Can you work these out from the model? Positions are in its coordinate system, mm. A direction names the side the tool comes from. Round coordinates to 2 decimals unless told otherwise and drop trailing zeros. Write each loop counter-clockwise with the first axis right and the second up, starting at its lowest first coordinate (ties: lowest second). Pieces come first, ordered by that corner, then holes. Notation, with made-up numbers: (19.5, -38.5) - (44.5, -38.5) arc R23 cw to (44.5, -18.5) - close; hole circle Ø2 at (-10, -29.5). An arc over 180 degrees is marked (long way). One line per item, written item: value. Start each with the question number.
(1) I want a section at A-A on z = 15.5. List the corners of the cut face in (x, y) for me (3 decimals).
(2) I want a section at C-C on x = 0. List the corners of the cut face in (y, z) for me, plus the area to 3 significant figures.
(3) Thinking about a two-plate mould opening in X: for faces 5 (the face through (32.96, 11.524, 18.645)), 6 (the face through (16, 30, 25)), 7 (the face through (26.46, -22.78, 18.64)), which applies, +X half, -X half, draft (parallel to the pull), parting line (faces both ways), or undercut?
(4) If I drill on L1, parallel to X at y = 0, z = 19.25; L2, parallel to X at y = 3.5, z = 6.5, over which ranges is the centre line in solid material (lowest first)? Write a range as from..to.
(5) I'm going to push flat-ended pins straight in: pin 1 Ø1 at (x, z) = (-8, 6.5) entering from -Y; pin 2 Ø8.5 at (x, y) = (-1.5, 34) entering from +Z; pin 3 Ø1.5 at (x, y) = (27.5, 6.5) entering from +Z. Where does each tip first touch, or does it pass through?
(6) On a 3-axis mill with a long thin cutter (end or side, diameter ignored), from which of +Z, -Z, +X, -X, +Y, -Y can I reach the whole of each face in a straight line? I mean faces 1 (the face through (0, 35, 12.109)), 2 (the face through (-26.46, 22.78, 18.64)), 3 (the face through (-33.084, 11.595, 18.645)), 4 (the face through (26.58, 22.85, 18.64)). Say none if no direction works.
(7) I want a section at B-B on y = 0. List the corners of the cut face in (x, z) for me, plus the area to 3 significant figures.
(8) I want a section at D-D on z = -1.5. List the corners of the cut face in (x, y) for me.
from build123d import *

# Parameters (mm, degrees)
F0_R            = 40
F0_R_2          = 30
F1_DEPTH        = 25
F3_DEPTH        = 12.8905829042
F3_COPIES_COUNT = 6
F5_R            = 40
F5_R_2          = 30
F6_DEPTH        = 5.8128256351


# Not quite as in the source:
# - a pattern or mirror of a feature is missing from the dataset's text; its kind, count and spacing are read off the source's solid


with BuildPart() as f1:
    # F0 (on Top) → F1 (new body)
    with BuildSketch(Plane.XY):
        Circle(F0_R)
        Circle(F0_R_2, mode=Mode.SUBTRACT)
    extrude(amount=F1_DEPTH)

    # F2 (on face) → F3 (cut)
    with BuildSketch(Plane.XY.offset(25)):
        with BuildLine():
            Line((6.5, 29.2873692912), (6.5, 39.4683417437))
            ThreePointArc((6.5, 39.4683417437), (3.2608534351, 39.8668638706), (0, 40))
            ThreePointArc((0, 40), (-3.2608534351, 39.8668638706), (-6.5, 39.4683417437))
            Line((-6.5, 39.4683417437), (-6.5, 29.2873692912))
            ThreePointArc((-6.5, 29.2873692912), (-3.2694740604, 29.8213101551), (0, 30))
            ThreePointArc((0, 30), (3.2694740604, 29.8213101551), (6.5, 29.2873692912))
        make_face()
    f3 = extrude(amount=-F3_DEPTH, mode=Mode.SUBTRACT)

    # F3_copies: F3 ×6 about axis
    f3_copies_axis = Axis((0, 0, 0), (0, 0, 1))
    for i in range(1, F3_COPIES_COUNT):
        add(f3.rotate(f3_copies_axis, i * 360 / F3_COPIES_COUNT), mode=Mode.SUBTRACT)

    # F5 (on face) → F6 (join)
    with BuildSketch(Plane(origin=(0, 0, 0), x_dir=(1, 0, 0), z_dir=(0, 0, -1))):
        Circle(F5_R)
        Circle(F5_R_2, mode=Mode.SUBTRACT)
        Circle(F5_R)
    extrude(amount=F6_DEPTH)


solid = f1.part
Established:
1. outline: (-37.431, -14.105) - (-28.614, -9.015) arc R30 cw to (-28.614, 9.015) - (-37.431, 14.105) arc R40 ccw to start; (-30.931, -25.363) arc R40 ccw to (-6.5, -39.468) - (-6.5, -29.287) arc R30 cw to (-22.114, -20.273) - close; (-30.931, 25.363) - (-22.114, 20.273) arc R30 cw to (-6.5, 29.287) - (-6.5, 39.468) arc R40 ccw to start; (6.5, -39.468) arc R40 ccw to (30.931, -25.363) - (22.114, -20.273) arc R30 cw to (6.5, -29.287) - close; (6.5, 29.287) arc R30 cw to (22.114, 20.273) - (30.931, 25.363) arc R40 ccw to (6.5, 39.468) - close; (28.614, -9.015) - (37.431, -14.105) arc R40 ccw to (37.431, 14.105) - (28.614, 9.015) arc R30 cw to start
2. outline: (-40, -5.81) - (40, -5.81) - (40, 12.11) - (30, 12.11) - (30, 0) - (-30, 0) - (-30, 12.11) - (-40, 12.11) - close
2. area: 707 mm2
3. face 5: undercut
3. face 6: draft
3. face 7: +X half
4. L1: -40..-30, 30..40
4. L2: -39.85..-29.8, 29.8..39.85
5. pin 1: y = -39.29
5. pin 2: z = 12.11
5. pin 3: z = 0
6. face 1: +Z, +Y, -Y
6. face 2: +Z, -X
6. face 3: +Z
6. face 4: +Z, +X
7. outline: (-40, -5.81) - (40, -5.81) - (40, 25) - (30, 25) - (30, 0) - (-30, 0) - (-30, 25) - (-40, 25) - close
7. area: 965 mm2
8. outline: circle Ø80 at (0, 0)
